```python
from build123d import *

# Parameters (mm, degrees)
ESQUISSE1_R        = 2
ESQUISSE1_R_2      = 1.6
ESQUISSE1_R_3      = 1.15
BOSS_EXTRU_1_DEPTH = 5
CONG_1_R           = 16
CONG_2_R           = 5


with BuildPart() as part:
    # Esquisse1 → Boss.-Extru.1 (new body)
    with BuildSketch(Plane.XY):
        with BuildLine():
            Line((-41.789550091, 25.514872575), (-67.043743505, 34.718675909))
            ThreePointArc((-67.043743505, 34.718675909), (75.07344073, -8.014268337), (-72.8619706, -19.783408206))
            Line((-72.8619706, -19.783408206), (-13.85803971, -32.618894281))
            Line((-13.85803971, -32.618894281), (1.569593433, 9.712782871))
            Line((1.569593433, 9.712782871), (-22.998575873, 18.666567095))
            Line((-22.998575873, 18.666567095), (-24.710652243, 13.96882354))
            Line((-24.710652243, 13.96882354), (-29.408395797, 15.68089991))
            Line((-29.408395797, 15.68089991), (-27.696319427, 20.378643465))
            Line((-27.696319427, 20.378643465), (-30.51496556, 21.405889287))
            Line((-30.51496556, 21.405889287), (-29.487719738, 24.224535419))
            Line((-29.487719738, 24.224535419), (-28.078396672, 23.710912508))
            Line((-28.078396672, 23.710912508), (-27.05115085, 26.529558641))
            Line((-27.05115085, 26.529558641), (-28.460473916, 27.043181552))
            Line((-28.460473916, 27.043181552), (-27.09081282, 30.801376396))
            Line((-27.09081282, 30.801376396), (-30.849007664, 32.171037492))
            Line((-30.849007664, 32.171037492), (-32.21866876, 28.412842648))
            Line((-32.21866876, 28.412842648), (-33.627991826, 28.926465559))
            Line((-33.627991826, 28.926465559), (-34.655237648, 26.107819426))
            Line((-34.655237648, 26.107819426), (-33.245914582, 25.594196515))
            Line((-33.245914582, 25.594196515), (-34.273160404, 22.775550383))
            Line((-34.273160404, 22.775550383), (-37.091806536, 23.802796205))
            Line((-37.091806536, 23.802796205), (-38.803882906, 19.10505265))
            Line((-38.803882906, 19.10505265), (-43.501626461, 20.81712902))
            Line((-43.501626461, 20.81712902), (-41.789550091, 25.514872575))
        make_face()
        with Locations((40.905825418, 50.514487495)):
            Circle(ESQUISSE1_R, mode=Mode.SUBTRACT)
        with Locations((-50.514487495, 40.905825418)):
            Circle(ESQUISSE1_R, mode=Mode.SUBTRACT)
        with Locations((50.514487495, -40.905825418)):
            Circle(ESQUISSE1_R, mode=Mode.SUBTRACT)
        with Locations((-40.905825418, -50.514487495)):
            Circle(ESQUISSE1_R, mode=Mode.SUBTRACT)
        with Locations((-28.497621404, 48.673941395)):
            Circle(ESQUISSE1_R_2, mode=Mode.SUBTRACT)
        with Locations((5.702522929, 56.11370803)):
            Circle(ESQUISSE1_R_2, mode=Mode.SUBTRACT)
        with Locations((5.702522929, -56.11370803)):
            Circle(ESQUISSE1_R_2, mode=Mode.SUBTRACT)
        with Locations((-28.497621404, -48.673941395)):
            Circle(ESQUISSE1_R_2, mode=Mode.SUBTRACT)
        with Locations((53.619184968, 17.5)):
            Circle(ESQUISSE1_R_2, mode=Mode.SUBTRACT)
        with Locations((53.619184968, -17.5)):
            Circle(ESQUISSE1_R_2, mode=Mode.SUBTRACT)
        with Locations((16.019184968, -17.5)):
            Circle(ESQUISSE1_R_2, mode=Mode.SUBTRACT)
        with Locations((16.019184968, 17.5)):
            Circle(ESQUISSE1_R_2, mode=Mode.SUBTRACT)
        with Locations((10.777554407, 0)):
            Circle(ESQUISSE1_R_3, mode=Mode.SUBTRACT)
        with Locations((34.819184968, 24.04163056)):
            Circle(ESQUISSE1_R_3, mode=Mode.SUBTRACT)
        with Locations((58.860815528, 0)):
            Circle(ESQUISSE1_R_3, mode=Mode.SUBTRACT)
        with Locations((34.819184968, -24.04163056)):
            Circle(ESQUISSE1_R_3, mode=Mode.SUBTRACT)
        with BuildLine():
            Line((-23.015077869, 35.23215147), (-23.440207391, 37.186445432))
            ThreePointArc((-23.440207391, 37.186445432), (-23.16841991, 38.692857499), (-21.911042951, 39.565868916))
            Line((-21.911042951, 39.565868916), (3.494778553, 45.092552701))
            ThreePointArc((3.494778553, 45.092552701), (5.00119062, 44.82076522), (5.874202037, 43.563388261))
            Line((5.874202037, 43.563388261), (6.299331559, 41.6090943))
            ThreePointArc((6.299331559, 41.6090943), (6.027544078, 40.102682233), (4.770167119, 39.229670816))
            Line((4.770167119, 39.229670816), (-20.635654385, 33.70298703))
            ThreePointArc((-20.635654385, 33.70298703), (-22.142066452, 33.974774511), (-23.015077869, 35.23215147))
        make_face(mode=Mode.SUBTRACT)
        with BuildLine():
            Line((6.299331559, -41.6090943), (5.874202037, -43.563388261))
            ThreePointArc((5.874202037, -43.563388261), (5.00119062, -44.82076522), (3.494778553, -45.092552701))
            Line((3.494778553, -45.092552701), (-21.911042951, -39.565868916))
            ThreePointArc((-21.911042951, -39.565868916), (-23.16841991, -38.692857499), (-23.440207391, -37.186445432))
            Line((-23.440207391, -37.186445432), (-23.015077869, -35.23215147))
            ThreePointArc((-23.015077869, -35.23215147), (-22.142066452, -33.974774511), (-20.635654385, -33.70298703))
            Line((-20.635654385, -33.70298703), (4.770167119, -39.229670816))
            ThreePointArc((4.770167119, -39.229670816), (6.027544078, -40.102682233), (6.299331559, -41.6090943))
        make_face(mode=Mode.SUBTRACT)
        with BuildLine():
            Line((39.319184968, 15), (41.319184968, 15))
            ThreePointArc((41.319184968, 15), (42.73339853, 14.414213562), (43.319184968, 13))
            Line((43.319184968, 13), (43.319184968, -13))
            ThreePointArc((43.319184968, -13), (42.73339853, -14.414213562), (41.319184968, -15))
            Line((41.319184968, -15), (39.319184968, -15))
            ThreePointArc((39.319184968, -15), (37.904971405, -14.414213562), (37.319184968, -13))
            Line((37.319184968, -13), (37.319184968, 13))
            ThreePointArc((37.319184968, 13), (37.904971405, 14.414213562), (39.319184968, 15))
        make_face(mode=Mode.SUBTRACT)
        with BuildLine():
            Line((30.319184968, -15), (28.319184968, -15))
            ThreePointArc((28.319184968, -15), (26.904971405, -14.414213562), (26.319184968, -13))
            Line((26.319184968, -13), (26.319184968, 13))
            ThreePointArc((26.319184968, 13), (26.904971405, 14.414213562), (28.319184968, 15))
            Line((28.319184968, 15), (30.319184968, 15))
            ThreePointArc((30.319184968, 15), (31.73339853, 14.414213562), (32.319184968, 13))
            Line((32.319184968, 13), (32.319184968, -13))
            ThreePointArc((32.319184968, -13), (31.73339853, -14.414213562), (30.319184968, -15))
        make_face(mode=Mode.SUBTRACT)
    extrude(amount=BOSS_EXTRU_1_DEPTH)

    # Congé1
    cong_1_edges = [part.edges().sort_by_distance(p)[0] for p in [
        (-72.8619706, -19.783408206, 2.5),
    ]]
    fillet(cong_1_edges, radius=CONG_1_R)

    # Congé2
    cong_2_edges = [part.edges().sort_by_distance(p)[0] for p in [
        (-67.043743505, 34.718675909, 2.5),
    ]]
    fillet(cong_2_edges, radius=CONG_2_R)


solid = part.part
```
Model file for the job. Use its own axes, mm. A direction names the side the tool comes from. Round coordinates to 2 decimals unless told otherwise and drop trailing zeros. Write each loop counter-clockwise with the first axis right and the second up, starting at its lowest first coordinate (ties: lowest second). Pieces come first, ordered by that corner, then holes. Notation, with made-up numbers: (-28.75, 85.25) - (11.25, 85.25) arc R8 cw to (11.25, 99.25) - close; hole circle Ø10 at (75.25, 48). An arc over 180 degrees is marked (long way). Use CSV: the item, a comma, the result in double quotes. Start each with the question number.
Item 1: Tool access for faces 5 (the face through (-51.497, 29.053, 2.465)), 6 (the face through (-9.39, 42.29, 2.46)): list every direction of +Z, -Z, +X, -X, +Y, -Y with a clear straight run to the whole face (end or side of a thin tool).
Item 2: Two-plate mould, pull along X, no slides. Class faces 1 (the face through (6, 1, 5)), 2 (the face through (-27.785, 28.896, 2.465)), 3 (the face through (-64.517, 35.822, 2.535)), 4 (the face through (15.811, -15.914, 2.465)): released by +X, released by -X, zero draft, split by the parting line, or undercut.
Item 3: Pin check, flat tips, straight feed: P1, Ø1.6, axis at x = 29, z = 3.5, coming from the +Y side; P2, Ø1, axis at x = 43, z = 1.5, coming from the +Y side; P3, Ø2, axis at x = 40, z = 3, coming from the -Y side. Stop position of each tip, or through.
Item 4: Drill centre lines: L1, parallel to X at y = -9.5, z = 1.4; L2, parallel to X at y = -6.5, z = 0.8; L3, parallel to Y at x = 2, z = 0.75. Where is each one in solid material? Low to high. Write a range as [from, to].
Item 5: Band-saw the part on A-A (y = -5). Write the cut outline in (x, z).
Item 6: Band-saw the part on C-C (x = 24). Write the cut outline in (y, z).
Item 7: Band-saw the part on B-B (z = 2.45). State how many separate pieces and enclosed holes the cut face has, and give its area (3 significant figures).
Checked values:
1,face 5,"+Z, -Z, -X"
1,face 6,"+Z, -Z"
2,face 1,"zero draft"
2,face 2,"undercut"
2,face 3,"released by -X"
2,face 4,"undercut"
3,P1,"stops at y = 70.04"
3,P2,"stops at y = 62.4"
3,P3,"stops at y = -64.65"
4,L1,"x = [-5.43, 26.32], [32.32, 37.32], [43.32, 74.9]"
4,L2,"x = [-4.34, 26.32], [32.32, 37.32], [43.32, 75.22]"
4,L3,"y = [-75.47, -44.77], [-38.63, 38.63], [44.77, 75.47]"
5,outline,"(-3.79, 0) - (26.32, 0) - (26.32, 5) - (-3.79, 5) - close; (32.32, 0) - (37.32, 0) - (37.32, 5) - (32.32, 5) - close; (43.32, 0) - (75.33, 0) - (75.33, 5) - (43.32, 5) - close"
6,outline,"(-71.58, 0) - (71.58, 0) - (71.58, 5) - (-71.58, 5) - close"
7,separate pieces,"1"
7,enclosed holes,"20"
7,area,"13,200 mm²"
